Read the model definition and answer for the solid it produces. Units are mm, in the model's axes. Coordinates: 2 decimals unless noted, no trailing zeros. Order: outer loops, then holes, each group sorted by start corner. A loop starts at its lowest first (then second) coordinate and runs counter-clockwise, first axis right, second up. Notation, with made-up numbers: M 21.5,79 L 76.5,79 A10 ccw 76.5,86 Z; hole C -21,80.25 d11. An arc over 180 degrees is marked long. Write each question's results on one line, items separated by ' | '.
```python
from build123d import *

# Parameters (mm, degrees)
SKETCH_1_R             = 2
SKETCH_1_R_2           = 4.25
SKETCH_1_R_3           = 1.5
SM_BASE_FLANGE_1_DEPTH = 3


# Sheet-metal steps are written as plain solids
with BuildPart() as part:
    # Sketch 1 → 基体-法兰1 (new body)
    with BuildSketch(Plane(origin=(0, 0, 0), x_dir=(1, 0, 0), z_dir=(0, 1, 0))):
        with BuildLine():
            Line((-80, 82.5), (80, 82.5))
            ThreePointArc((80, 82.5), (87.071067812, 79.571067812), (90, 72.5))
            Line((90, 72.5), (90, -72.5))
            ThreePointArc((90, -72.5), (87.071067812, -79.571067812), (80, -82.5))
            Line((80, -82.5), (-80, -82.5))
            ThreePointArc((-80, -82.5), (-87.071067812, -79.571067812), (-90, -72.5))
            Line((-90, -72.5), (-90, 72.5))
            ThreePointArc((-90, 72.5), (-87.071067812, 79.571067812), (-80, 82.5))
        make_face()
        with Locations(Location((0, 72.5, 0), (0, 0, 270))):
            Circle(SKETCH_1_R, mode=Mode.SUBTRACT)
        with Locations(Location((60, 72.5, 0), (0, 0, 270))):
            Circle(SKETCH_1_R, mode=Mode.SUBTRACT)
        with Locations(Location((-60, 72.5, 0), (0, 0, 270))):
            Circle(SKETCH_1_R, mode=Mode.SUBTRACT)
        with Locations(Location((0, -72.5, 0), (0, 0, 270))):
            Circle(SKETCH_1_R, mode=Mode.SUBTRACT)
        with Locations(Location((-60, -72.5, 0), (0, 0, 270))):
            Circle(SKETCH_1_R, mode=Mode.SUBTRACT)
        with Locations(Location((60, -72.5, 0), (0, 0, 270))):
            Circle(SKETCH_1_R, mode=Mode.SUBTRACT)
        with Locations(Location((0, 37.5, 0), (0, 0, 270))):
            Circle(SKETCH_1_R_2, mode=Mode.SUBTRACT)
        with Locations(Location((18.5, 37.5, 0), (0, 0, 270))):
            Circle(SKETCH_1_R, mode=Mode.SUBTRACT)
        with Locations(Location((-18.5, 37.5, 0), (0, 0, 270))):
            Circle(SKETCH_1_R, mode=Mode.SUBTRACT)
        with Locations(Location((70, 52.5, 0), (0, 0, 270))):
            Circle(SKETCH_1_R_3, mode=Mode.SUBTRACT)
        with Locations(Location((70, 0, 0), (0, 0, 270))):
            Circle(SKETCH_1_R_3, mode=Mode.SUBTRACT)
        with Locations(Location((70, -52.5, 0), (0, 0, 270))):
            Circle(SKETCH_1_R_3, mode=Mode.SUBTRACT)
        with Locations(Location((-70, 52.5, 0), (0, 0, 270))):
            Circle(SKETCH_1_R_3, mode=Mode.SUBTRACT)
        with Locations(Location((-70, 0, 0), (0, 0, 270))):
            Circle(SKETCH_1_R_3, mode=Mode.SUBTRACT)
        with Locations(Location((-70, -52.5, 0), (0, 0, 270))):
            Circle(SKETCH_1_R_3, mode=Mode.SUBTRACT)
        with Locations(Location((0, -52.5, 0), (0, 0, 270))):
            Circle(SKETCH_1_R_3, mode=Mode.SUBTRACT)
    extrude(amount=-SM_BASE_FLANGE_1_DEPTH)


solid = part.part
```
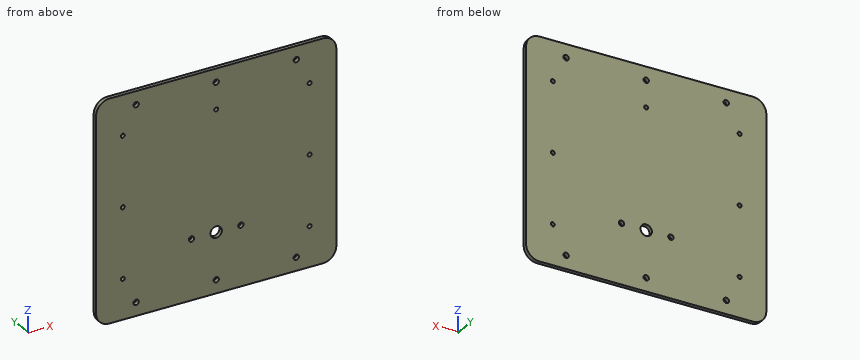
(1) Given pin 1 (2.5 mm diameter, centred on x = -70, z = 0, fed in from +Y), flat-ended and moving along its own axis, determine where the tip first touches the part or whether it passes through.
Conclusion:
pin 1: through
(2) Straight lines are drawn through the part: line 1 (X direction, y = -1.35, z = -52.5); line 2 (Z direction, x = 70, y = -1.4); line 3 (X direction, y = -2.2, z = -72.5). For each, find the intervals that lie inside material, in ascending order.
Conclusion:
line 1: -90 to -71.5, -68.5 to 68.5, 71.5 to 90 | line 2: -82.5 to -54, -51 to -1.5, 1.5 to 51, 54 to 82.5 | line 3: -90 to -62, -58 to -2, 2 to 58, 62 to 90
(3) The part is cut by section A-A, the plane z = -37.5. Write down the section's boundary in (x, y), then the cut area to 4 significant figures.
Conclusion:
outline: M -90,-3 L -20.5,-3 L -20.5,0 L -90,0 Z; M -16.5,-3 L -4.25,-3 L -4.25,0 L -16.5,0 Z; M 4.25,-3 L 16.5,-3 L 16.5,0 L 4.25,0 Z; M 20.5,-3 L 90,-3 L 90,0 L 20.5,0 Z | area: 490.5 mm²
